Autodesk Inventor part; units mm, degrees
ref_plane "YZ Plane" through (0, 0, 0) normal (1, 0, 0) x (0, 1, 0)
ref_plane "XZ Plane" through (0, 0, 0) normal (0, 1, 0) x (-1, 0, 0)
ref_plane "XY Plane" through (0, 0, 0) normal (0, 0, 1) x (1, 0, 0)
sketch "Sketch1" plane through (0, 0, 0) normal (0, 0, 1) x (1, 0, 0)
  circle A0 centre (0, 0) radius 9.5
  dimension "d0" = 19
extrude "Extrusion1" add sketch "Sketch1" along normal blind 440
hole "Hole1" at (0, 0, 440) direction (0, 0, -1) diameter 10 depth 70 tip angle 118
hole "Hole2" at (0, 0, 0) direction (0, 0, 1) diameter 10 depth 70 tip angle 118
properties part number "Barra-garfo" material "Aluminium AW-7020"
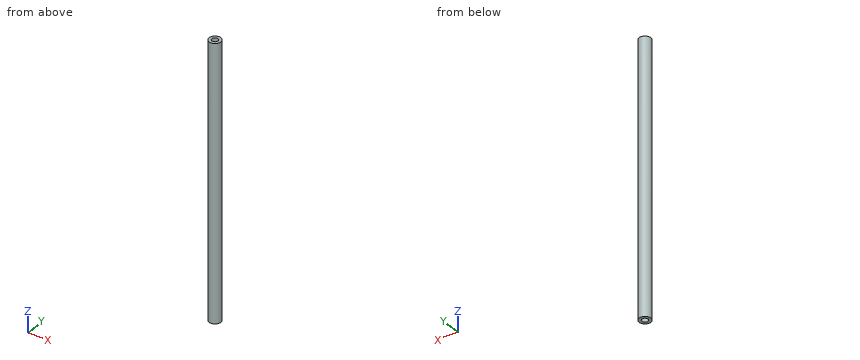
Design review of the part built by this model. Coordinates are the model's own, in mm. Round coordinates to 2 decimals unless told otherwise and drop trailing zeros. Order: outer loops, then holes, each group sorted by start corner. A loop starts at its lowest first (then second) coordinate and runs counter-clockwise, first axis right, second up. Notation, with made-up numbers: (-14.5, 57.5) - (35.5, 57.5) arc R24 cw to (35.5, 77.5) - close; hole circle Ø10 at (-25.75, -35.75). An arc over 180 degrees is marked (long way). One line per question, with ' | ' between items.
Item 1: Take a section at A-A, the plane z = 51. Write out the cut boundary in (x, y), then the cut area to 3 significant figures.
Checks:
outline: circle Ø19 at (0, 0); hole circle Ø10 at (0, 0) | area: 205 mm²
Item 2: Wall thickness on line 1 (Y direction, x = 0, z = 392); line 2 (X direction, y = -0.25, z = 411); line 3 (X direction, y = -3.25, z = 382): over which ranges is each line inside the solid? List them lowest first. Write a range as [from, to].
Checks:
line 1: [-9.5, -5], [5, 9.5] | line 2: [-9.5, -4.99], [4.99, 9.5] | line 3: [-8.93, -3.8], [3.8, 8.93]
Item 3: Take a section at B-B, the plane z = 138. Write out the cut boundary in (x, y).
Checks:
outline: circle Ø19 at (0, 0)
Item 4: For P1, Ø4, axis at y = -4, z = 205, coming from the +X side; P2, Ø8, axis at y = 7, z = 52, coming from the +X side; P3, Ø8, axis at x = 0, y = 0, coming from the -Z side, all flat-tipped, find the tip position at first contact; note any pin that passes through.
Checks:
P1: x = 9.29 | P2: x = 9.01 | P3: z = 70.6
